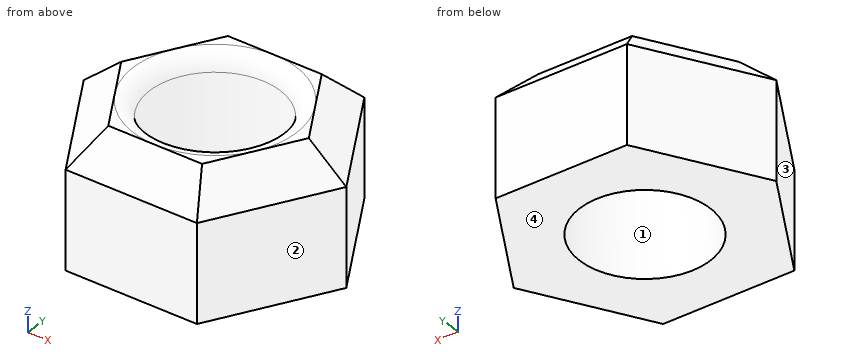
Autodesk Inventor part; units mm, degrees
ref_plane "YZ Plane" through (0, 0, 0) normal (1, 0, 0) x (0, 1, 0)
ref_plane "XZ Plane" through (0, 0, 0) normal (0, 1, 0) x (-1, 0, 0)
ref_plane "XY Plane" through (0, 0, 0) normal (0, 0, 1) x (1, 0, 0)
sketch "Sketch1" plane through (0, 0, 0) normal (0, 0, 1) x (1, 0, 0)
  circle A0 centre (0, 0) radius 3.175
  line L0 (3.2079, 5.5562) -> (6.4158, 0)
  line L1 (6.4158, 0) -> (3.2079, -5.5563)
  line L2 (3.2079, -5.5563) -> (-3.2079, -5.5562)
  line L3 (-3.2079, -5.5562) -> (-6.4158, 0)
  line L4 (-6.4158, 0) -> (-3.2079, 5.5562)
  line L5 (-3.2079, 5.5562) -> (3.2079, 5.5562)
  dimension "d0" = 6.35
  dimension "d1" = 11.1125
extrude "Extrusion1" add sketch "Sketch1" along normal blind 6.35
chamfer "Chamfer1" distance 1.5875 angle 45 6 edges at (4.8119, 2.7781, 6.35) (0, 5.5562, 6.35) (-4.8119, 2.7781, 6.35) (-4.8119, -2.7781, 6.35) (0, -5.5563, 6.35) (4.8119, -2.7781, 6.35)
thread "Thread1"
fillet "Fillet1" radius 0.7937 1 edges at (-3.175, 0, 6.35)
properties part number "nut_.25_20"
Geometry: final body of the model. Coordinates: model frame, mm. Face numbers are marked on the shaded views. Coordinates: 2 decimals unless noted, no trailing zeros. Write each loop counter-clockwise with the first axis right and the second up, starting at its lowest first coordinate (ties: lowest second). Pieces come first, ordered by that corner, then holes. Notation, with made-up numbers: M 86,68.25 L 122,68.25 A30 ccw 122,91.25 Z; hole C 35,52 d11. An arc over 180 degrees is marked long. Use CSV: the item, a comma, the result in double quotes. Start each with the question number.
1. First-contact query: P1, Ø6, axis at x = 4, y = 1, coming from the -Z side; P2, Ø1, axis at y = -3, z = 5, coming from the -X side; P3, Ø3, axis at x = -2, y = 1, coming from the +Z side; P4, Ø4, axis at x = 1, y = -1, coming from the +Z side. Flat tips, straight axial feed; report the tip coordinate or a pass-through.
2. Cut plane C-C on z = 5.25. Return the cut outline in (x, y) (3 decimals).
3. Mould query, pull axis X, two halves, no side actions, for the marked faces 1, 2, 3 and 4. Classes: pulls with the +X half, pulls with the -X half, needs draft (parallel to the pull), parting line crosses it, or undercut.
4. Cut plane A-A on z = 0.5. Return the cut outline in (x, y) (3 decimals).
5. Ray query, probe 1 along Y at (x, z) = (0, 2.3) (3 decimals); probe 2 along X at (y, z) = (0.5, 2); probe 3 along X at (y, z) = (-0.75, 1.25). Return the intervals inside material, ascending.
Entries:
1,P1,"z = 0"
1,P2,"x = -4.94"
1,P3,"z = 6.32"
1,P4,"z = 6.12"
2,outline,"M -5.853,0 L -2.926,-5.069 L 2.926,-5.069 L 5.853,0 L 2.926,5.069 L -2.926,5.069 Z; hole C 0,0 d6.35"
3,face 1,"undercut"
3,face 2,"pulls with the +X half"
3,face 3,"pulls with the -X half"
3,face 4,"needs draft"
4,outline,"M -6.416,0 L -3.208,-5.556 L 3.208,-5.556 L 6.416,0 L 3.208,5.556 L -3.208,5.556 Z; hole C 0,0 d6.35"
5,probe 1,"-5.556 to -3.175, 3.175 to 5.556"
5,probe 2,"-6.13 to -3.14, 3.14 to 6.13"
5,probe 3,"-5.98 to -3.09, 3.09 to 5.98"
